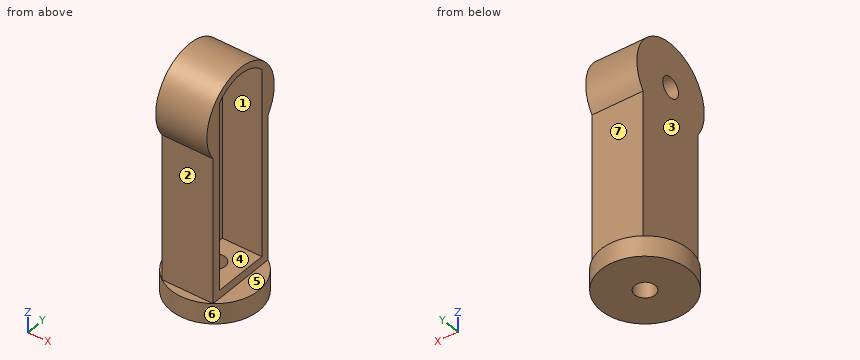
from build123d import *

# Parameters (mm, degrees)
CROQUIS2_R              = 21.5
CROQUIS2_R_2            = 5
CROQUIS2_W              = 71.010004003
CROQUIS2_H              = 35
SALIENTE_EXTRUIR1_DEPTH = 12.5
CORTAR_EXTRUIR1_DEPTH   = 19.2
CROQUIS4_R              = 21.5
SALIENTE_EXTRUIR2_DEPTH = 10
CROQUIS5_R              = 5
CORTAR_EXTRUIR3_DEPTH   = 19


with BuildPart() as part:
    # Croquis2 → Saliente-Extruir1 (new, symmetric)
    # profile 1 of 2: a face of its own
    with BuildSketch(Plane(origin=(0, 0, 0), x_dir=(0, 0, -1), z_dir=(1, 0, 0))):
        with Locations((-24.062155912, 0)):
            Circle(CROQUIS2_R)
        with Locations((-24.062155912, 0)):
            Circle(CROQUIS2_R_2, mode=Mode.SUBTRACT)
    # profile 2 of 2: a face of its own
    with BuildSketch(Plane(origin=(0, 0, 0), x_dir=(0, 0, -1), z_dir=(1, 0, 0))):
        with Locations((23.932842087, 0)):
            Rectangle(CROQUIS2_W, CROQUIS2_H)
    extrude(amount=SALIENTE_EXTRUIR1_DEPTH, both=True)

    # Croquis3 → Cortar-Extruir1 (cut)
    with BuildSketch(Plane(origin=(12.5, 0, 0), x_dir=(0, 0, -1), z_dir=(1, 0, 0))):
        with BuildLine():
            Line((55.437844088, -13.5), (55.437844088, 13.5))
            Line((55.437844088, 13.5), (-11.739767465, 13.5))
            ThreePointArc((-11.739767465, 13.5), (-7.339089709, 7.377690276), (-5.783992518, 0))
            ThreePointArc((-5.783992518, 0), (-7.339089709, -7.377690276), (-11.739767465, -13.5))
            Line((-11.739767465, -13.5), (55.437844088, -13.5))
        make_face()
        with BuildLine():
            ThreePointArc((-5.783992518, 0), (-7.339089709, 7.377690276), (-11.739767465, 13.5))
            Line((-11.739767465, 13.5), (-36.384544359, 13.5))
            Line((-36.384544359, 13.5), (-36.384544359, -13.5))
            Line((-36.384544359, -13.5), (-11.739767465, -13.5))
            ThreePointArc((-11.739767465, -13.5), (-7.339089709, -7.377690276), (-5.783992518, 0))
        make_face()
        with BuildLine():
            Line((-36.384544359, -13.5), (-36.384544359, 13.5))
            ThreePointArc((-36.384544359, 13.5), (-42.340319305, 0), (-36.384544359, -13.5))
        make_face()
    extrude(amount=-CORTAR_EXTRUIR1_DEPTH, mode=Mode.SUBTRACT)

    # Croquis4 → Saliente-Extruir2 (add)
    with BuildSketch(Plane(origin=(0, 0, -59.437844088), x_dir=(-1, 0, 0), z_dir=(0, 0, -1))):
        with Locations(Location((0, 0, 0), (0, 0, 125.548744003))):
            Circle(CROQUIS4_R)
    extrude(amount=SALIENTE_EXTRUIR2_DEPTH)

    # Croquis5 → Cortar-Extruir3 (cut)
    with BuildSketch(Plane(origin=(0, 0, -69.437844088), x_dir=(-1, 0, 0), z_dir=(0, 0, -1))):
        Circle(CROQUIS5_R)
    extrude(amount=-CORTAR_EXTRUIR3_DEPTH, mode=Mode.SUBTRACT)


solid = part.part
CAD build for the part. Positions are in the model's coordinates, mm. Face numbers are marked on the shaded views. A direction names the side the tool comes from. Give positions to 0.01 mm unless a question says otherwise; leave off trailing zeros. Loops run counter-clockwise (first coordinate to the right, second up) from the corner with the lowest first, then second, coordinate; pieces in that order, holes last. Notation, with made-up numbers: M 39,50.5 L 66,50.5 A38 cw 66,89.5 Z; hole C 54,77 d5. An arc over 180 degrees is marked long. One line per question, with ' | ' between items. Start each with the question number.
1. Two-plate mould, pull along Y, no slides. Class the marked faces 1, 2, 3 and 4: pulls with the +Y half, pulls with the -Y half, needs draft (parallel to the pull), parting line crosses it, or undercut.
2. Saw through at D-D on z = 28. Give the cut face in (x, y).
3. 3-axis set-ups, long thin cutter, end or side, ignore diameter. For the marked faces 5, 6 and 7: which of +Z, -Z, +X, -X, +Y, -Y reach the whole face in a straight line?
4. Flat gauge pins, fed straight in: pin 1 (21 mm diameter, centred on x = 5.5, y = -3, fed in from +Z); pin 2 (6 mm diameter, centred on x = -15, z = -28.5, fed in from +Y); pin 3 (4 mm diameter, centred on x = -16, z = -25.5, fed in from +Y); pin 4 (5 mm diameter, centred on x = -11.5, z = 33.5, fed in from -Y). Where does each tip first touch, or does it go through?
5. Probe L1, parallel to Z at x = -9.6, y = 0; L2, parallel to Y at x = 0, z = -62.5; L3, parallel to Y at x = 6.5, z = -30. List the from-to ranges inside material, lowest first. Write a range as from..to.
6. Saw through at C-C on x = 0. Give the cut face in (y, z), plus the area to 3 significant figures.
7. Saw through at B-B on z = -13.5. Give the cut face in (x, y).
8. Saw through at A-A on y = 0. Give the cut face in (x, z), plus the area to 3 significant figures.
Result sheet:
1) face 1: undercut | face 2: pulls with the -Y half | face 3: needs draft | face 4: undercut
2) outline: M -12.5,-21.14 L 12.5,-21.14 L 12.5,-13.5 L -6.7,-13.5 L -6.7,-3.08 L -12.5,-3.08 Z; M -12.5,3.08 L -6.7,3.08 L -6.7,13.5 L 12.5,13.5 L 12.5,21.14 L -12.5,21.14 Z
3) face 5: +Z, +X, +Y, -Y | face 6: -Z | face 7: +X, -X, +Y
4) pin 1: stops at z = 45.56 | pin 2: stops at y = 17.5 | pin 3: passes through | pin 4: stops at y = -20.35
5) L1: z = -69.44..19.06, 29.06..45.56 | L2: y = -21.5..-5, 5..21.5 | L3: y = -17.5..-13.5, 13.5..17.5
6) outline: M -21.5,-69.44 L -5,-69.44 L -5,-55.44 L -13.5,-55.44 L -13.5,36.38 A18.28 cw 13.5,36.38 L 13.5,-55.44 L 5,-55.44 L 5,-69.44 L 21.5,-69.44 L 21.5,-59.44 L 17.5,-59.44 L 17.5,11.57 A21.5 ccw long -17.5,11.57 L -17.5,-59.44 L -21.5,-59.44 Z | area: 1,420 mm^2
7) outline: M -12.5,-17.5 L 12.5,-17.5 L 12.5,-13.5 L -6.7,-13.5 L -6.7,13.5 L 12.5,13.5 L 12.5,17.5 L -12.5,17.5 Z
8) outline: M -21.5,-69.44 L -5,-69.44 L -5,-55.44 L -6.7,-55.44 L -6.7,19.06 L -12.5,19.06 L -12.5,-59.44 L -21.5,-59.44 Z; M -12.5,29.06 L -6.7,29.06 L -6.7,42.34 L 12.5,42.34 L 12.5,45.56 L -12.5,45.56 Z; M 5,-69.44 L 21.5,-69.44 L 21.5,-59.44 L 12.5,-59.44 L 12.5,-55.44 L 5,-55.44 Z | area: 980 mm^2
